Build history of the part. All positions in model axes, mm. Face numbers are marked on the shaded views. A direction names the side the tool comes from. Round coordinates to 2 decimals unless told otherwise and drop trailing zeros. Write each loop counter-clockwise with the first axis right and the second up, starting at its lowest first coordinate (ties: lowest second). Pieces come first, ordered by that corner, then holes.
1) Saw through at A-A (z = 12.7). State how many separate pieces and enclosed holes the cut face has, plus the area to 3 significant figures.
2) Wall check: probe 1 along Y at (x, z) = (44, 16.25); probe 2 along X at (y, z) = (6.75, 20); probe 3 along Y at (x, z) = (20.5, 12.7). Give the ranges that are in metal, low to high.
3) Which spindle directions (+Z, -Z, +X, -X, +Y, -Y) get a long thin tool onto all of the face, cutting with end or side? Do the marked faces 4, 5, 6, 7 and 8. Say none if no direction does.
4) Flat gauge pins, fed straight in: pin 1 (4.5 mm diameter, centred on y = 8, z = 2, fed in from -X); pin 2 (6 mm diameter, centred on x = 31, z = 22.5, fed in from -Y); pin 3 (1.5 mm diameter, centred on y = 10, z = 20, fed in from +X); pin 4 (10 mm diameter, centred on x = 57.15, z = 12.7, fed in from +Y). Where does each tip first touch, or does it go through?
5) Saw through at C-C (x = 31.75). Write the cut outline in (y, z) (3 decimals), plus the area to 3 significant figures.
6) Saw through at B-B (y = 4.25). Write the cut outline in (x, z) (3 decimals).
7) Pull direction Z, two halves, no side cores. Call the marked faces 1, 2 and 3: +Z half, -Z half, draft (parallel to the pull), parting line (faces both ways), or undercut.
from build123d import *

# Parameters (mm, degrees)
BOSS_EXTRUDE1_DEPTH          = 25.4
F_1_2_0_75_DIAMETER_HOLE2_D  = 19.05
F_1_2_0_25_DIAMETER_HOLE1_D  = 6.35
F_1_2_0_25_DIAMETER_HOLE2_D  = 6.35
F_1_2_0_375_DIAMETER_HOLE1_D = 9.525


with BuildPart() as part:
    # Sketch1 → Boss-Extrude1 (new body)
    with BuildSketch(Plane.XY):
        Polygon((0, 0), (25.4, 0), (25.4, 12.7), (38.1, 12.7), (38.1, 0), (69.85, 0), (69.85, 6.35), (44.45, 6.35), (44.45, 19.05), (19.05, 19.05), (19.05, 6.35), (0, 6.35), align=None)
    extrude(amount=BOSS_EXTRUDE1_DEPTH)

    # 1/2 (0.75) Diameter Hole2 (through all)
    with Locations(Plane(origin=(0, 19.05, 0), x_dir=(1, 0, 0), z_dir=(0, 1, 0))):
        with Locations((31.75, -12.7)):
            Hole(F_1_2_0_75_DIAMETER_HOLE2_D / 2)

    # 1/2 (0.25) Diameter Hole1 (through all)
    with Locations(Plane(origin=(0, 6.35, 0), x_dir=(1, 0, 0), z_dir=(0, 1, 0))):
        with Locations((9.525, -12.7)):
            Hole(F_1_2_0_25_DIAMETER_HOLE1_D / 2)

    # 1/2 (0.25) Diameter Hole2 (through all)
    with Locations(Plane(origin=(0, 6.35, 0), x_dir=(1, 0, 0), z_dir=(0, 1, 0))):
        with Locations((57.15, -12.7)):
            Hole(F_1_2_0_25_DIAMETER_HOLE2_D / 2)

    # 1/2 (0.375) Diameter Hole1 (through all)
    with Locations(Plane(origin=(44.45, 0, 0), x_dir=(0, 0, -1), z_dir=(1, 0, 0))):
        with Locations((-12.7, 12.7)):
            Hole(F_1_2_0_375_DIAMETER_HOLE1_D / 2)


solid = part.part
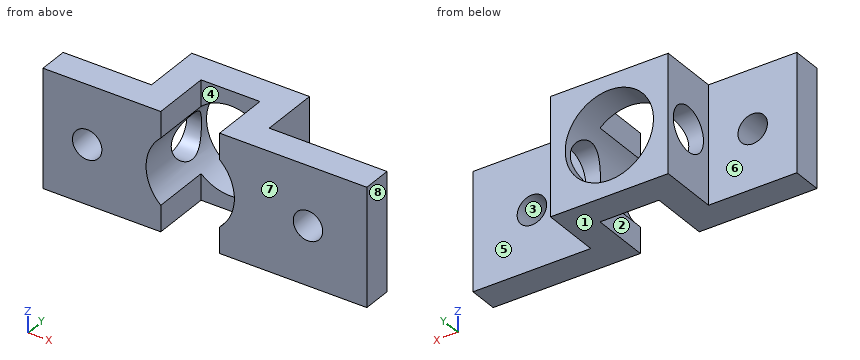
Evaluation:
1. separate pieces: 6
1. enclosed holes: 0
1. area: 262 mm2
2. probe 1: y = 0 to 9.53, 15.87 to 19.05
2. probe 2: x = 19.05 to 25.4, 38.1 to 44.45
2. probe 3: y = 0 to 7.94, 17.46 to 19.05
3. face 4: +Z, -Z, -Y
3. face 5: +Z, -Z, +X, +Y
3. face 6: +Z, -Z, -X, +Y
3. face 7: +Z, -Z, +X, -X, -Y
3. face 8: +Z, -Z, +X, +Y, -Y
4. pin 1: stops at x = 0
4. pin 2: stops at y = 12.7
4. pin 3: stops at x = 44.45
4. pin 4: stops at y = 6.35
5. outline: (12.7, 0) - (19.05, 0) - (19.05, 3.175) - (12.7, 3.175) - close; (12.7, 22.225) - (19.05, 22.225) - (19.05, 25.4) - (12.7, 25.4) - close
5. area: 40.3 mm2
6. outline: (0, 0) - (25.4, 0) - (25.4, 5.6) arc R9.525 cw to (25.4, 19.8) - (25.4, 25.4) - (0, 25.4) - close; (38.1, 0) - (69.85, 0) - (69.85, 25.4) - (38.1, 25.4) - (38.1, 19.8) arc R9.525 cw to (38.1, 5.6) - close; hole circle Ø6.35 at (9.525, 12.7); hole circle Ø6.35 at (57.15, 12.7)
7. face 1: -Z half
7. face 2: draft
7. face 3: undercut
